Input: part model. Units: mm. Frame: model coordinates. A direction names the side the tool comes from. Coordinates: 2 decimals unless noted, no trailing zeros. Write each loop counter-clockwise with the first axis right and the second up, starting at its lowest first coordinate (ties: lowest second). Pieces come first, ordered by that corner, then holes. Notation, with made-up numbers: (87.5, -37.5) -> (104.5, -37.5) arc R18 cw to (104.5, -11.5) -> close; hole circle Ø1 at (-22, -18). An arc over 180 degrees is marked (long way). Use one line per item in the form item = value. Start each with the question number.
(1) First-contact query: pin 1 (11 mm diameter, centred on y = -80, z = 98, fed in from +X); pin 2 (24.5 mm diameter, centred on x = -1, y = -15, fed in from +Z); pin 3 (8 mm diameter, centred on x = 0, y = -1.5, fed in from +Z). Flat tips, straight axial feed; report the tip coordinate or a pass-through.
(2) Cut plane C-C on x = 26.5. State how many separate pieces and enclosed holes the cut face has, plus the area to 3 significant figures.
(3) Cut plane A-A on x = 0. Return the cut outline in (y, z), plus the area to 3 significant figures.
(4) Cut plane D-D on y = -66.5. Return the cut outline in (x, z), plus the area to 3 significant figures.
(5) Ray query, line 1 along X through (y, z) = (-6, 135); line 2 along Y through (x, z) = (-0.5, -22.5). Return the intervals inside material, ascending.
(6) Pull-direction query (Y, two-part tool) for faces 6 (the face through (0, 0, 140)), 7 (the face through (-0.595, 16.839, 64.517)), 8 (the face through (-0.867, 21.538, 61.595)); classes: released by +Y, released by -Y, zero draft, split by the parting line, or undercut.
(7) Set-up query: faces 1 (the face through (-39.7, 9.3, 58)), 2 (the face through (26.53, -29.26, 75.47)), 3 (the face through (0, -7, 136)), 4 (the face through (-1, 11, 66)), 5 (the face through (42.75, -79, 101)). Return all of +Z, -Z, +X, -X, +Y, -Y with unobstructed straight access to the full face (end or side cutting, diameter ignored); none if empty.
(8) Cut plane B-B on z = 38. Return the cut outline in (x, y), plus the area to 3 significant figures.
```python
from build123d import *

# Parameters (mm, degrees)
SKETCH1_R           = 41
BOSS_EXTRUDE1_DEPTH = 62
SKETCH2_R           = 41
BOSS_EXTRUDE2_DEPTH = 4
SKETCH3_R           = 41
SKETCH3_R_2         = 40.5
CUT_EXTRUDE1_DEPTH  = 8
SKETCH5_R           = 10.75
BOSS_EXTRUDE3_DEPTH = 70
SKETCH6_R           = 5
BOSS_EXTRUDE4_DEPTH = 4
BOSS_EXTRUDE5_DEPTH = 10.75
SKETCH8_R           = 7
BOSS_EXTRUDE6_DEPTH = 32
SKETCH9_R           = 12
BOSS_EXTRUDE7_DEPTH = 45
SKETCH10_R          = 4.75
BOSS_EXTRUDE8_DEPTH = 23.5


with BuildPart() as part:
    # Sketch1 → Boss-Extrude1 (new, symmetric)
    with BuildSketch(Plane.XY):
        Circle(SKETCH1_R)
    extrude(amount=BOSS_EXTRUDE1_DEPTH, both=True)

    # Sketch2 → Boss-Extrude2 (add, symmetric)
    with BuildSketch(Plane.XY.offset(62)):
        Circle(SKETCH2_R)
    extrude(amount=BOSS_EXTRUDE2_DEPTH, both=True)

    # Sketch3 → Cut-Extrude1 (cut)
    with BuildSketch(Plane.XY.offset(66)):
        Circle(SKETCH3_R)
        Circle(SKETCH3_R_2, mode=Mode.SUBTRACT)
    extrude(amount=-CUT_EXTRUDE1_DEPTH, mode=Mode.SUBTRACT)

    # Sketch4 → Cut-Revolve1 (revolve, cut)
    with BuildSketch(Plane(origin=(0, 0, 0), x_dir=(0, 0, -1), z_dir=(1, 0, 0)), mode=Mode.PRIVATE) as cut_revolve1_sk:
        with BuildLine():
            Line((-58, 41), (-61.774006584, 20.588938621))
            ThreePointArc((-61.774006584, 20.588938621), (-62.166989532, 19.454504548), (-62.878908123, 18.487784224))
            Line((-62.878908123, 18.487784224), (-64.828427125, 16.538265222))
            ThreePointArc((-64.828427125, 16.538265222), (-66.12612052, 15.671174217), (-67.656854249, 15.366692347))
            Line((-67.656854249, 15.366692347), (-68, 15.366692347))
            Line((-68, 15.366692347), (-68, 44))
            Line((-68, 44), (-58, 44))
            Line((-58, 44), (-58, 41))
        make_face()
    revolve(cut_revolve1_sk.sketch.rotate(Axis((0, 0, 0), (0, 0, -1)), 90), axis=Axis((0, 0, 0), (0, 0, -1)), mode=Mode.SUBTRACT)

    # Sketch5 → Boss-Extrude3 (add)
    with BuildSketch(Plane.XY.offset(66)):
        Circle(SKETCH5_R)
    extrude(amount=BOSS_EXTRUDE3_DEPTH)

    # Sketch6 → Boss-Extrude4 (add, symmetric)
    with BuildSketch(Plane.XY.offset(136)):
        Circle(SKETCH6_R)
    extrude(amount=BOSS_EXTRUDE4_DEPTH, both=True)

    # Sketch7 → Boss-Extrude5 (add, symmetric)
    with BuildSketch(Plane(origin=(0, 0, 0), x_dir=(0, 0, -1), z_dir=(1, 0, 0))):
        with BuildLine():
            Line((-136, 0), (-136, -17.890978608))
            ThreePointArc((-136, -17.890978608), (-114.282888831, -83.926914424), (-58.092450033, -43))
            Line((-58.092450033, -43), (-58.092450033, 0))
            Line((-58.092450033, 0), (-136, 0))
        make_face()
    extrude(amount=BOSS_EXTRUDE5_DEPTH, both=True)

    # Sketch8 → Boss-Extrude6 (add)
    with BuildSketch(Plane(origin=(10.75, 0, 0), x_dir=(0, 0, -1), z_dir=(1, 0, 0))):
        with Locations((-69.915535496, -25)):
            Circle(SKETCH8_R)
        with Locations(Location((-101.092450033, -79, 0), (0, 0, 269.999665288))):
            Circle(SKETCH8_R)
        with Locations(Location((-132.269364569, -25, 0), (0, 0, 149.999665321))):
            Circle(SKETCH8_R)
    extrude(amount=BOSS_EXTRUDE6_DEPTH)

    # Sketch9 → Boss-Extrude7 (add)
    with BuildSketch(Plane(origin=(10.75, 0, 0), x_dir=(0, 0, -1), z_dir=(1, 0, 0))):
        with Locations(Location((-101.092450033, -43, 0), (0, 0, 180))):
            Circle(SKETCH9_R)
    extrude(amount=BOSS_EXTRUDE7_DEPTH)

    # Sketch10 → Boss-Extrude8 (add)
    with BuildSketch(Plane(origin=(55.75, 0, 0), x_dir=(0, 0, -1), z_dir=(1, 0, 0))):
        with Locations((-101.092450033, -43)):
            Circle(SKETCH10_R)
    extrude(amount=BOSS_EXTRUDE8_DEPTH)


solid = part.part
```
Values:
q1.pin_1 = 42.75
q1.pin_2 = 141.1
q1.pin_3 = 140
q2.separate_pieces = 5
q2.enclosed_holes = 0
q2.area = 8,530 mm2
q3.outline = (-43, 58.09) -> (-40.5, 58.09) -> (-40.5, 58) -> (-41, 58) -> (-41, -62) -> (41, -62) -> (41, 58) -> (40.5, 58) -> (40.5, 58.09) -> (20.59, 61.77) arc R4 cw to (18.49, 62.88) -> (16.54, 64.83) arc R4 cw to (15.73, 66) -> (10.75, 66) -> (10.75, 136) -> (5, 136) -> (5, 140) -> (-5, 140) -> (-5, 136) -> (-17.89, 136) arc R43 ccw (long way) to start
q3.area = 17,200 mm2
q4.outline = (-10.75, 65.08) -> (10.75, 65.08) -> (10.75, 137.1) -> (-10.75, 137.1) -> close
q4.area = 1,550 mm2
q5.line_1 = -10.75 to 10.75
q5.line_2 = -41 to 41
q6.face_6 = zero draft
q6.face_7 = undercut
q6.face_8 = split by the parting line
q7.face_1 = none
q7.face_2 = +X
q7.face_3 = +Z
q7.face_4 = +Z, +Y
q7.face_5 = +Z, -Z, +X, -Y
q8.outline = circle Ø82 at (0, 0)
q8.area = 5,280 mm2
